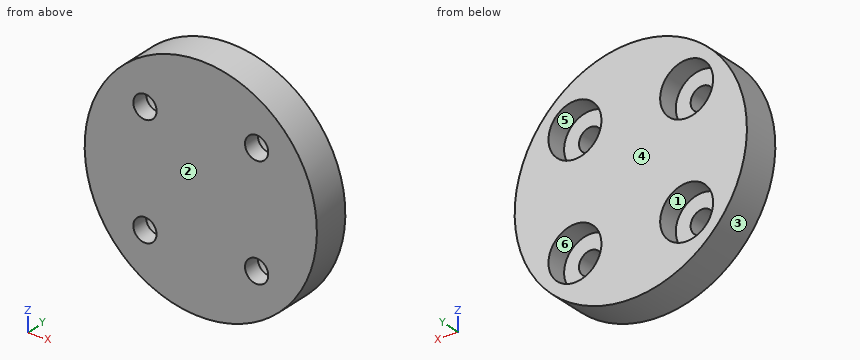
from build123d import *

# Parameters (mm, degrees)
SKETCH_1_R          = 12.5
EXTRUDE_1_DEPTH     = 4
SKETCH_2_R          = 2.85
CUT_EXTRUDE_1_DEPTH = 2.2
SKETCH_3_R          = 1.25
CUT_EXTRUDE_2_DEPTH = 10


with BuildPart() as part:
    # 草图1 → 凸台-拉伸1 (new body)
    with BuildSketch(Plane(origin=(0, 0, 0), x_dir=(1, 0, 0), z_dir=(0, 1, 0))):
        with Locations(Location((0, 0, 0), (0, 0, 270))):
            Circle(SKETCH_1_R)
    extrude(amount=EXTRUDE_1_DEPTH)

    # 草图2 → 切除-拉伸1 (cut)
    with BuildSketch(Plane(origin=(0, 4, 0), x_dir=(1, 0, 0), z_dir=(0, 1, 0))):
        with Locations(Location((6.01040764, 6.01040764, 0), (0, 0, 270))):
            Circle(SKETCH_2_R)
        with Locations(Location((6.01040764, -6.01040764, 0), (0, 0, 270))):
            Circle(SKETCH_2_R)
        with Locations(Location((-6.01040764, -6.01040764, 0), (0, 0, 270))):
            Circle(SKETCH_2_R)
        with Locations(Location((-6.01040764, 6.01040764, 0), (0, 0, 270))):
            Circle(SKETCH_2_R)
    extrude(amount=-CUT_EXTRUDE_1_DEPTH, mode=Mode.SUBTRACT)

    # 草图3 → 切除-拉伸2 (cut)
    with BuildSketch(Plane(origin=(0, 1.8, 0), x_dir=(1, 0, 0), z_dir=(0, 1, 0))):
        with Locations(Location((-6.01040764, 6.01040764, 0), (0, 0, 270))):
            Circle(SKETCH_3_R)
        with Locations(Location((6.01040764, 6.01040764, 0), (0, 0, 270))):
            Circle(SKETCH_3_R)
        with Locations(Location((6.01040764, -6.01040764, 0), (0, 0, 270))):
            Circle(SKETCH_3_R)
        with Locations(Location((-6.01040764, -6.01040764, 0), (0, 0, 270))):
            Circle(SKETCH_3_R)
    extrude(amount=-CUT_EXTRUDE_2_DEPTH, mode=Mode.SUBTRACT)


solid = part.part
Design review of the part built by this model. Coordinates are the model's own, in mm. Face numbers are marked on the shaded views. A direction names the side the tool comes from. Give positions to 0.01 mm unless a question says otherwise; leave off trailing zeros. Loops run counter-clockwise (first coordinate to the right, second up) from the corner with the lowest first, then second, coordinate; pieces in that order, holes last. Notation, with made-up numbers: M -17.75,46 L -9.75,46 A26 cw -9.75,82 Z; hole C 30.5,75 d3. An arc over 180 degrees is marked long. Write item = value, one per line.
Q1. We need section D-D (z = 8.5). Give the boundary of the cut face in (x, y).
Output values:
outline = M -9.17,0 L 9.17,0 L 9.17,4 L 7.4,4 L 7.4,1.8 L 4.62,1.8 L 4.62,4 L -4.62,4 L -4.62,1.8 L -7.4,1.8 L -7.4,4 L -9.17,4 Z
Q2. Insertion check: pin 1 (2 mm diameter, centred on y = 2.5, z = -1.5, fed in from -X); pin 2 (3 mm diameter, centred on x = -6, z = -6.5, fed in from +Y); pin 3 (1.5 mm diameter, centred on y = 3, z = 6.5, fed in from +X). Each pin has a flat end and moves straight along its axis. Give the tip position at first contact, or say it passes through.
Output values:
pin_1 = -12.49
pin_2 = 1.8
pin_3 = 11.1
Q3. We need section B-B (y = 0.85). Give the boundary of the cut face in (x, z), plus the area to 3 significant figures.
Output values:
outline = C 0,0 d25; hole C -6.01,-6.01 d2.5; hole C -6.01,6.01 d2.5; hole C 6.01,-6.01 d2.5; hole C 6.01,6.01 d2.5
area = 471 mm^2
Q4. We need section A-A (z = -6). Give the boundary of the cut face in (x, y), plus the area to 3 significant figures.
Output values:
outline = M -10.97,0 L -7.26,0 L -7.26,1.8 L -8.86,1.8 L -8.86,4 L -10.97,4 Z; M -4.76,0 L 4.76,0 L 4.76,1.8 L 3.16,1.8 L 3.16,4 L -3.16,4 L -3.16,1.8 L -4.76,1.8 Z; M 7.26,0 L 10.97,0 L 10.97,4 L 8.86,4 L 8.86,1.8 L 7.26,1.8 Z
area = 53.6 mm^2
Q5. Draft analysis for pull direction Z (two halves, no side actions). For the marked faces 3, 4, 5 and 6, state which applies: +Z half, -Z half, draft (parallel to the pull), parting line (faces both ways), or undercut.
Output values:
face_3 = parting line
face_4 = draft
face_5 = undercut
face_6 = undercut
Q6. To check wall thickness, follow line 1 (Z direction, x = -3.5, y = 2.55); line 2 (X direction, y = 1.9, z = 6.5); line 3 (X direction, y = 1.9, z = -4.5). State the ranges of each line that lie inside material, in increasing order. Write a range as [from, to].
Output values:
line_1 = [-12, -7.36], [-4.66, 4.66], [7.36, 12]
line_2 = [-10.68, -8.82], [-3.2, 3.2], [8.82, 10.68]
line_3 = [-11.66, -8.43], [-3.59, 3.59], [8.43, 11.66]
Q7. We need section C-C (x = 7.75). Give the boundary of the cut face in (y, z).
Output values:
outline = M 0,-9.81 L 4,-9.81 L 4,-8.27 L 1.8,-8.27 L 1.8,-3.75 L 4,-3.75 L 4,3.75 L 1.8,3.75 L 1.8,8.27 L 4,8.27 L 4,9.81 L 0,9.81 Z
Q8. For the marked faces 1 and 2, list the 3-axis set-ups (+Z, -Z, +X, -X, +Y, -Y) from which the entire face can be reached by the end or side of a thin tool; tool diameter is ignored.
Output values:
face_1 = +Y
face_2 = +Z, -Z, +X, -X, -Y
